```python
from build123d import *

# Parameters (mm, degrees)
SKETCH1_W                                   = 95
SKETCH1_H                                   = 30
BOSS_EXTRUDE1_DEPTH                         = 90
F_2_MM_TOP_BOT_3_MM_SIDE_T                  = -3
F_2_MM_TOP_BOT_3_MM_SIDE_THICKNESS_2_FACE_W = 84
F_2_MM_TOP_BOT_3_MM_SIDE_THICKNESS_2_FACE_H = 27
F_2_MM_TOP_BOT_3_MM_SIDE_THICKNESS_2_DEPTH  = 2
F_2_MM_TOP_BOT_3_MM_SIDE_THICKNESS_3_FACE_W = 84
F_2_MM_TOP_BOT_3_MM_SIDE_THICKNESS_3_FACE_H = 27
F_2_MM_TOP_BOT_3_MM_SIDE_THICKNESS_3_DEPTH  = 2
SKETCH4_R                                   = 3.55
F_7_1_MM_FIXTURE_HOLES_DEPTH                = 10
F_5_MM_RADIUS_R                             = 5
CUT_EXTRUDE1_DEPTH                          = 10


with BuildPart() as part:
    # Sketch1 → Boss-Extrude1 (new body)
    with BuildSketch(Plane(origin=(0, 0, 0), x_dir=(0, 1, 0), z_dir=(0, 0, 1))):
        Rectangle(SKETCH1_W, SKETCH1_H)
    extrude(amount=BOSS_EXTRUDE1_DEPTH)

    # 2 mm top/bot 3 mm side
    f_2_mm_top_bot_3_mm_side_openings = [part.faces().sort_by_distance(p)[0] for p in [
        (-15, 0, 45),
    ]]
    offset(amount=F_2_MM_TOP_BOT_3_MM_SIDE_T, openings=f_2_mm_top_bot_3_mm_side_openings, kind=Kind.INTERSECTION)

    # 2 mm top/bot 3 mm side thickness 2 face (on inner face of the shell) → 2 mm top/bot 3 mm side thickness 2 (add)
    with BuildSketch(Plane(origin=(-1.5, 44.5, 45), x_dir=(0, 0, 1), z_dir=(0, 1, 0))):
        Rectangle(F_2_MM_TOP_BOT_3_MM_SIDE_THICKNESS_2_FACE_W, F_2_MM_TOP_BOT_3_MM_SIDE_THICKNESS_2_FACE_H)
    extrude(amount=-F_2_MM_TOP_BOT_3_MM_SIDE_THICKNESS_2_DEPTH)

    # 2 mm top/bot 3 mm side thickness 3 face (on inner face of the shell) → 2 mm top/bot 3 mm side thickness 3 (add)
    with BuildSketch(Plane(origin=(-1.5, -44.5, 45), x_dir=(0, 0, -1), z_dir=(0, -1, 0))):
        Rectangle(F_2_MM_TOP_BOT_3_MM_SIDE_THICKNESS_3_FACE_W, F_2_MM_TOP_BOT_3_MM_SIDE_THICKNESS_3_FACE_H)
    extrude(amount=-F_2_MM_TOP_BOT_3_MM_SIDE_THICKNESS_3_DEPTH)

    # Sketch4 → 7.1 mm fixture holes (cut)
    with BuildSketch(Plane.XY.offset(90)):
        with Locations((0, 24.2)):
            Circle(SKETCH4_R)
        Circle(SKETCH4_R)
        with Locations((0, -24.2)):
            Circle(SKETCH4_R)
        with BuildLine():
            ThreePointArc((0, -3.55), (-3.55, 0), (0, 3.55))
            Line((0, 3.55), (-15, 3.55))
            Line((-15, 3.55), (-15, -3.55))
            Line((-15, -3.55), (0, -3.55))
        make_face()
    extrude(amount=-F_7_1_MM_FIXTURE_HOLES_DEPTH, mode=Mode.SUBTRACT)

    # 5 mm radius
    f_5_mm_radius_edges = [part.edges().sort_by_distance(p)[0] for p in [
        (0, 47.5, 90),
        (12, 0, 3),
        (12, -42.5, 45),
        (-1.5, 42.5, 3),
        (12, 42.5, 45),
        (-1.5, -42.5, 87),
        (12, 0, 87),
        (-1.5, 42.5, 87),
        (-1.5, -42.5, 3),
        (0, -47.5, 90),
        (15, 0, 90),
        (0, -47.5, 0),
        (0, 47.5, 0),
        (15, 0, 0),
        (15, -47.5, 45),
        (15, 47.5, 45),
    ]]
    fillet(f_5_mm_radius_edges, radius=F_5_MM_RADIUS_R)

    # Sketch3 → Cut-Extrude1 (cut)
    with BuildSketch(Plane(origin=(0, 0, 0), x_dir=(1, 0, 0), z_dir=(0, 0, -1))):
        with BuildLine():
            ThreePointArc((5, 32.5), (3.535533906, 36.035533906), (0, 37.5))
            Line((0, 37.5), (0, 27.5))
            ThreePointArc((0, 27.5), (3.535533906, 28.964466094), (5, 32.5))
        make_face()
        with BuildLine():
            Line((0, 27.5), (0, 37.5))
            ThreePointArc((0, 37.5), (-5, 32.5), (0, 27.5))
        make_face()
        with BuildLine():
            ThreePointArc((5, 12.5), (3.535533906, 16.035533906), (0, 17.5))
            Line((0, 17.5), (0, 7.5))
            ThreePointArc((0, 7.5), (3.535533906, 8.964466094), (5, 12.5))
        make_face()
        with BuildLine():
            Line((0, 7.5), (0, 17.5))
            ThreePointArc((0, 17.5), (-5, 12.5), (0, 7.5))
        make_face()
        with BuildLine():
            ThreePointArc((5, -7.5), (3.535533906, -3.964466094), (0, -2.5))
            Line((0, -2.5), (0, -12.5))
            ThreePointArc((0, -12.5), (3.535533906, -11.035533906), (5, -7.5))
        make_face()
        with BuildLine():
            Line((0, -12.5), (0, -2.5))
            ThreePointArc((0, -2.5), (-5, -7.5), (0, -12.5))
        make_face()
        with BuildLine():
            ThreePointArc((5, -27.5), (3.535533906, -23.964466094), (0, -22.5))
            Line((0, -22.5), (0, -27.5))
            Line((0, -27.5), (0, -32.5))
            ThreePointArc((0, -32.5), (3.535533906, -31.035533906), (5, -27.5))
        make_face()
        with BuildLine():
            Line((0, -27.5), (0, -22.5))
            ThreePointArc((0, -22.5), (-5, -27.5), (0, -32.5))
            Line((0, -32.5), (0, -27.5))
        make_face()
    extrude(amount=-CUT_EXTRUDE1_DEPTH, mode=Mode.SUBTRACT)


solid = part.part
```
Work out the finished part from the listing and answer in its coordinate system (mm). A direction names the side the tool comes from. Give positions to 0.01 mm unless a question says otherwise; leave off trailing zeros. Order: outer loops, then holes, each group sorted by start corner. A loop starts at its lowest first (then second) coordinate and runs counter-clockwise, first axis right, second up. Notation, with made-up numbers: M -34.75,72.25 L -30.75,72.25 A25 cw -30.75,84.25 Z; hole C 73,54 d9. An arc over 180 degrees is marked long. Return JSON: item names as keys, results as strings.
1) For a pull along Z with two mould halves and no side action, classify faces 1 (the flat face through (15, -1, 44)), 2 (the cylindrical face through (10, 1, 4)), 3 (the cylindrical face through (-2.68, 46, 88.57)) as +Z half, -Z half, draft (parallel to the pull), parting line (faces both ways), or undercut.
Resolved:
{"face 1": "draft", "face 2": "undercut", "face 3": "+Z half"}
2) Straight lines are drawn through the part: line 1 along Y through (x, z) = (0, 88.6); line 2 along Y through (x, z) = (0, 88.5); line 3 along Y through (x, z) = (3, 19.5). For each, find the intervals that lie inside material, in ascending order. Write a range as [from, to].
Resolved:
{"line 1": "[-45.97, -27.75], [-20.65, -3.55], [3.55, 20.65], [27.75, 45.97]", "line 2": "[-46.07, -27.75], [-20.65, -3.55], [3.55, 20.65], [27.75, 46.07]", "line 3": "[-47.5, -42.5], [42.5, 47.5]"}
3) Section B-B, the plane x = -9.5 is taken. Write down the section's boundary in (y, z).
Resolved:
{"outline": "M -47.5,5 A5 ccw -42.5,0 L 42.5,0 A5 ccw 47.5,5 L 47.5,85 A5 ccw 42.5,90 L 3.55,90 L 3.55,87 L 37.5,87 A5 cw 42.5,82 L 42.5,8 A5 cw 37.5,3 L -37.5,3 A5 cw -42.5,8 L -42.5,82 A5 cw -37.5,87 L -3.55,87 L -3.55,90 L -42.5,90 A5 ccw -47.5,85 Z"}
4) Section C-C, the plane z = 12 is taken. Write down the section's boundary in (x, y).
Resolved:
{"outline": "M -15,-47.5 L 10,-47.5 A5 ccw 15,-42.5 L 15,42.5 A5 ccw 10,47.5 L -15,47.5 L -15,42.5 L 7,42.5 A5 cw 12,37.5 L 12,-37.5 A5 cw 7,-42.5 L -15,-42.5 Z"}
5) A tool of negligible diameter and unlimited length cuts with its end or side. For faces 4 (the cylindrical face through (-0.46, -20.68, 88.52)), 5 (the flat face through (-8, -3.55, 89)), 6 (the flat face through (12, -1, 44)), 7 (the cylindrical face through (-2.68, -46.07, 1.5)), 8 (the cylindrical face through (-2.68, -46, 88.57)), from which of +Z, -Z, +X, -X, +Y, -Y can it reach the whole face along a straight path? Write none if from no direction.
Resolved:
{"face 4": "+Z", "face 5": "+Z, -X", "face 6": "-X", "face 7": "-Z, +X, -X, -Y", "face 8": "+Z, +X, -X, -Y"}
6) Each of these flat-tipped pins is pushed along its axis until it touches: pin 1 (11.5 mm diameter, centred on x = 0, y = -24.2, fed in from -Z); pin 2 (3.5 mm diameter, centred on x = -8.5, z = 89, fed in from -Y); pin 3 (3.5 mm diameter, centred on x = -8, z = 88, fed in from +Y); pin 4 (10 mm diameter, centred on y = -19, z = 66.5, fed in from -X). Where does it stop, or does it pass through?
Resolved:
{"pin 1": "z = 0", "pin 2": "y = -46.97", "pin 3": "y = 47.34", "pin 4": "x = 12"}
7) Section D-D, the plane y = 24.2 is taken. Write down the section's boundary in (x, z).
Resolved:
{"outline": "M -15,0 L -3.76,0 L -3.76,3 L -15,3 Z; M -15,87 L -3.55,87 L -3.55,90 L -15,90 Z; M 3.55,87 L 7,87 A5 cw 12,82 L 12,8 A5 cw 7,3 L 3.76,3 L 3.76,0 L 10,0 A5 ccw 15,5 L 15,85 A5 ccw 10,90 L 3.55,90 Z"}
8) Section A-A, the plane y = -24.2 is taken. Write down the section's boundary in (x, z), plus the area to 3 significant figures.
Resolved:
{"outline": "M -15,0 L 10,0 A5 ccw 15,5 L 15,85 A5 ccw 10,90 L 3.55,90 L 3.55,87 L 7,87 A5 cw 12,82 L 12,8 A5 cw 7,3 L -15,3 Z; M -15,87 L -3.55,87 L -3.55,90 L -15,90 Z", "area": "411 mm^2"}
